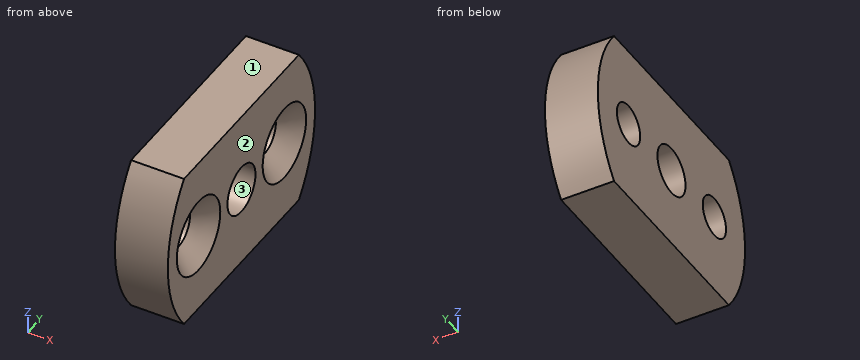
from build123d import *

# Parameters (mm, degrees)
SKETCH1_R                                      = 1.7272
SKETCH1_R_2                                    = 2.286
BOSS_EXTRUDE1_DEPTH                            = 4.953
CSK_FOR_6_FLAT_HEAD_MACHINE_SCREW1_D           = 3.7973
CSK_FOR_6_FLAT_HEAD_MACHINE_SCREW1_DEPTH       = 10.973
CSK_FOR_6_FLAT_HEAD_MACHINE_SCREW1_CSINK_D     = 7.0866
CSK_FOR_6_FLAT_HEAD_MACHINE_SCREW1_CSINK_ANGLE = 82
CSK_FOR_6_FLAT_HEAD_MACHINE_SCREW1_TIP         = 1.140824014


with BuildPart() as part:
    # Sketch1 → Boss-Extrude1 (new body)
    with BuildSketch(Plane(origin=(0, 0, 0), x_dir=(0, 0, -1), z_dir=(1, 0, 0))):
        with BuildLine():
            Line((-7.5, 9.367496998), (-7.5, -9.367496998))
            ThreePointArc((-7.5, -9.367496998), (0, -12), (7.5, -9.367496998))
            Line((7.5, -9.367496998), (7.5, 9.367496998))
            ThreePointArc((7.5, 9.367496998), (0, 12), (-7.5, 9.367496998))
        make_face()
        with Locations((0, 7)):
            Circle(SKETCH1_R, mode=Mode.SUBTRACT)
        with Locations((0, -7)):
            Circle(SKETCH1_R, mode=Mode.SUBTRACT)
        Circle(SKETCH1_R_2, mode=Mode.SUBTRACT)
    extrude(amount=BOSS_EXTRUDE1_DEPTH)

    # CSK for #6 Flat Head Machine Screw1
    with Locations(Plane(origin=(4.953, 0, 0), x_dir=(0, 0, -1), z_dir=(1, 0, 0))):
        with Locations((0, -7), (0, 7)):
            CounterSinkHole(CSK_FOR_6_FLAT_HEAD_MACHINE_SCREW1_D / 2, CSK_FOR_6_FLAT_HEAD_MACHINE_SCREW1_CSINK_D / 2, depth=CSK_FOR_6_FLAT_HEAD_MACHINE_SCREW1_DEPTH, counter_sink_angle=CSK_FOR_6_FLAT_HEAD_MACHINE_SCREW1_CSINK_ANGLE)
            with Locations((0, 0, -(CSK_FOR_6_FLAT_HEAD_MACHINE_SCREW1_DEPTH + CSK_FOR_6_FLAT_HEAD_MACHINE_SCREW1_TIP / 2))):  # 118° drill point
                Cone(0, CSK_FOR_6_FLAT_HEAD_MACHINE_SCREW1_D / 2, CSK_FOR_6_FLAT_HEAD_MACHINE_SCREW1_TIP, mode=Mode.SUBTRACT)


solid = part.part
Model file for the job. Use its own axes, mm. Face numbers are marked on the shaded views. Give positions to 0.01 mm unless a question says otherwise; leave off trailing zeros. Loops run counter-clockwise (first coordinate to the right, second up) from the corner with the lowest first, then second, coordinate; pieces in that order, holes last.
1) Saw through at D-D (y = 0). Write the cut outline in (x, z), plus the area to 4 significant figures.
2) Wall check: line 1 (Z direction, x = 2.4, y = -7); line 2 (Y direction, x = 4.3, z = -1.75); line 3 (Y direction, x = 3.1, z = -1). Give the ranges that are in metal, low to high.
3) Saw through at B-B (z = 0). Write the cut outline in (x, y).
4) Saw through at A-A (y = -7). Write the cut outline in (x, z), plus the area to 3 significant figures.
5) Saw through at C-C (x = 0.9). Write the cut outline in (y, z).
6) Pull direction Z, two halves, no side cores. Call the marked faces 1, 2 and 3: +Z half, -Z half, draft (parallel to the pull), parting line (faces both ways), or undercut.
7) Flat gauge pins, fed straight in: pin 1 Ø4 at (y, z) = (0, 0) entering from -X; pin 2 Ø1 at (x, z) = (2.5, -4.5) entering from +Y; pin 3 Ø6 at (y, z) = (7, -0.5) entering from +X. Where does each tip first touch, or does it go through?
Answer block:
1. outline: (0, -7.5) - (4.95, -7.5) - (4.95, -2.29) - (0, -2.29) - close; (0, 2.29) - (4.95, 2.29) - (4.95, 7.5) - (0, 7.5) - close
1. area: 51.65 mm2
2. line 1: z = -7.5 to -1.9, 1.9 to 7.5
2. line 2: y = -11.87 to -9.41, -4.59 to -1.47, 1.47 to 4.59, 9.41 to 11.87
2. line 3: y = -11.96 to -8.65, -5.35 to -2.06, 2.06 to 5.35, 8.65 to 11.96
3. outline: (0, -12) - (4.95, -12) - (4.95, -10.54) - (3.06, -8.9) - (0, -8.9) - close; (0, -5.1) - (3.06, -5.1) - (4.95, -3.46) - (4.95, -2.29) - (0, -2.29) - close; (0, 2.29) - (4.95, 2.29) - (4.95, 3.46) - (3.06, 5.1) - (0, 5.1) - close; (0, 8.9) - (3.06, 8.9) - (4.95, 10.54) - (4.95, 12) - (0, 12) - close
4. outline: (0, -7.5) - (4.95, -7.5) - (4.95, -3.54) - (3.06, -1.9) - (0, -1.9) - close; (0, 1.9) - (3.06, 1.9) - (4.95, 3.54) - (4.95, 7.5) - (0, 7.5) - close
4. area: 52.4 mm2
5. outline: (-9.37, -7.5) - (9.37, -7.5) arc R12 ccw to (9.37, 7.5) - (-9.37, 7.5) arc R12 ccw to start; hole circle Ø3.8 at (-7, 0); hole circle Ø4.57 at (0, 0); hole circle Ø3.8 at (7, 0)
6. face 1: +Z half
6. face 2: draft
6. face 3: undercut
7. pin 1: passes through
7. pin 2: stops at y = 11.31
7. pin 3: stops at x = 4.9
